Source: CAD feature listing. Evaluate the final solid. Frame: model axes, mm. Face numbers are marked on the shaded views. A direction names the side the tool comes from. Round coordinates to 2 decimals unless told otherwise and drop trailing zeros. Order: outer loops, then holes, each group sorted by start corner. A loop starts at its lowest first (then second) coordinate and runs counter-clockwise, first axis right, second up. Notation, with made-up numbers: (-13, 5.5) - (1, 5.5) arc R9 cw to (1, 16.5) - close; hole circle Ø8 at (-20.75, 18). An arc over 180 degrees is marked (long way). Use one line per item in the form item = value. Start each with the question number.
Q1. Cut plane A-A, the plane z = 4.25. Return the cut outline in (x, y).
Q2. Pin query (flat end, axial travel): pin 1 Ø0.8 at (x, z) = (4.5, 7.5) entering from +Y. Return the tip coordinate at first contact, or that it passes through.
Q3. Cut plane B-B, the plane y = 5.5. Return the cut outline in (x, z), and give its area (3 significant figures).
Q4. Set-up query: the marked faces 1 and 2. Return all of +Z, -Z, +X, -X, +Y, -Y with unobstructed straight access to the full face (end or side cutting, diameter ignored); none if empty.
Q5. Ray query, line 1 (X direction, y = 4.5, z = 5); line 2 (Y direction, x = 4.75, z = 2.75). Return the intervals inside material, ascending. Write a range as [from, to].
from build123d import *

# Parameters (mm, degrees)
PAD_DEPTH = 12
FILLET_R  = 0.5


with BuildPart() as part:
    # Sketch → Pad (new body)
    with BuildSketch(Plane.XY):
        Polygon((0, 0), (16, 0), (16, 7), (5, 7), (5, 4), (3.5, 4), (3.5, 7), (0, 7), align=None)
    extrude(amount=PAD_DEPTH)

    # Fillet
    fillet_edges = [part.edges().sort_by_distance(p)[0] for p in [
        (10.5, 7, 0),
        (16, 7, 6),
        (5, 7, 6),
        (10.5, 7, 12),
        (1.75, 7, 12),
        (0, 7, 6),
        (3.5, 7, 6),
        (1.75, 7, 0),
        (0, 3.5, 0),
        (16, 3.5, 0),
        (16, 3.5, 12),
        (0, 3.5, 12),
    ]]
    fillet(fillet_edges, radius=FILLET_R)


solid = part.part
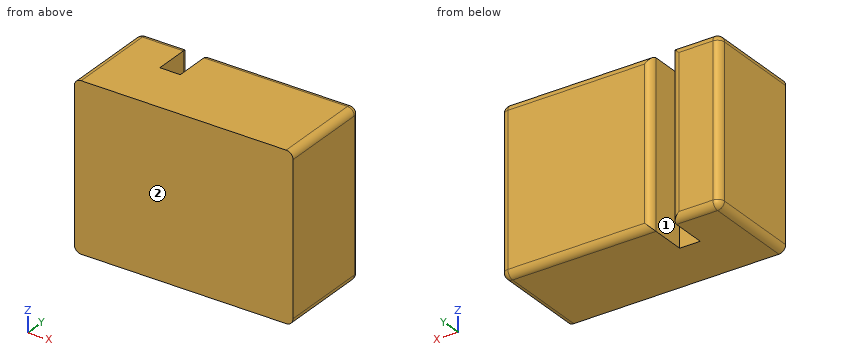
Completed:
q1.outline = (0, 0) - (16, 0) - (16, 6.5) arc R0.5 ccw to (15.5, 7) - (5.5, 7) arc R0.5 ccw to (5, 6.5) - (5, 4) - (3.5, 4) - (3.5, 6.5) arc R0.5 ccw to (3, 7) - (0.5, 7) arc R0.5 ccw to (0, 6.5) - close
q2.pin_1 = 4
q3.outline = (0, 0.5) arc R0.5 ccw to (0.5, 0) - (3.5, 0) - (3.5, 12) - (0.5, 12) arc R0.5 ccw to (0, 11.5) - close; (5, 0) - (15.5, 0) arc R0.5 ccw to (16, 0.5) - (16, 11.5) arc R0.5 ccw to (15.5, 12) - (5, 12) - close
q3.area = 174 mm2
q4.face_1 = +Z, -Z, +Y
q4.face_2 = +Z, -Z, +X, -X, -Y
q5.line_1 = [0, 3.5], [5, 16]
q5.line_2 = [0, 4]
